The model under review builds one solid part; all positions refer to its coordinate system, in mm. Face numbers are marked on the shaded views. A direction names the side the tool comes from. Give positions to 0.01 mm unless a question says otherwise; leave off trailing zeros. Write each loop counter-clockwise with the first axis right and the second up, starting at its lowest first coordinate (ties: lowest second). Pieces come first, ordered by that corner, then holes. Notation, with made-up numbers: (60.25, -13) -> (89.25, -13) arc R18 cw to (89.25, 11) -> close; hole circle Ø4 at (76, -10). An arc over 180 degrees is marked (long way). Use CSV: the item, a comma, the result in double quotes.
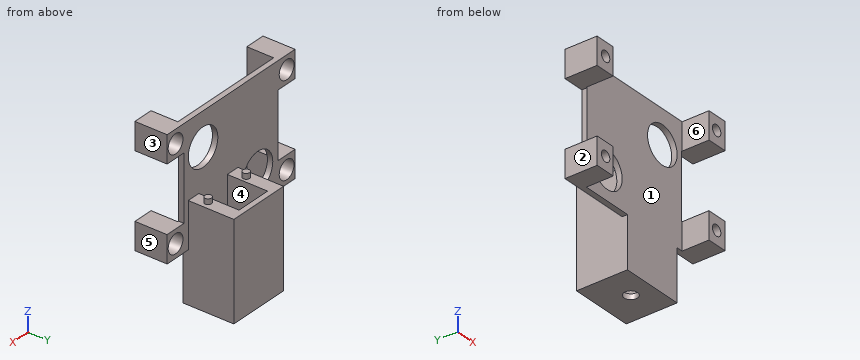
```python
from build123d import *

# Parameters (mm, degrees)
SKETCH_R        = 2
PAD_DEPTH       = 2
SKETCH001_W     = 7.6
SKETCH001_H     = 10.1
SKETCH001_R     = 2
PAD001_DEPTH    = 10
SKETCH002_R     = 7
POCKET_DEPTH    = 12.001
SKETCH004_W     = 13.5
SKETCH004_H     = 15
PAD003_DEPTH    = 34
SKETCH005_W     = 23.5
SKETCH005_H     = 19
SKETCH005_R     = 2.5
PAD004_DEPTH    = 2
SKETCH006_R     = 1.25
PAD005_DEPTH    = 2
SKETCH007_R     = 3.5
POCKET001_DEPTH = 5


with BuildPart() as part:
    # Sketch → Pad (new body)
    with BuildSketch(Plane.XZ):
        Polygon((-22.275, 22.25), (22.275, 22.25), (30.275, 22.25), (30.275, 12.15), (22.275, 12.15), (22.275, -12.15), (30.275, -12.15), (30.275, -22.25), (22.275, -22.25), (-22.275, -22.25), (-30.275, -22.25), (-30.275, -12.15), (-22.275, -12.15), (-22.275, 12.15), (-30.275, 12.15), (-30.275, 22.25), align=None)
        with Locations((-26.275, 17.2)):
            Circle(SKETCH_R, mode=Mode.SUBTRACT)
        with Locations((26.275, 17.2)):
            Circle(SKETCH_R, mode=Mode.SUBTRACT)
        with Locations((26.275, -17.2)):
            Circle(SKETCH_R, mode=Mode.SUBTRACT)
        with Locations((-26.275, -17.2)):
            Circle(SKETCH_R, mode=Mode.SUBTRACT)
    extrude(amount=PAD_DEPTH)

    # Sketch001 (on Face22 of Pad) → Pad001 (join)
    with BuildSketch(Plane.XZ.offset(2)):
        with Locations((-26.475, 17.2)):
            Rectangle(SKETCH001_W, SKETCH001_H)
        with Locations((-26.275, 17.2)):
            Circle(SKETCH001_R, mode=Mode.SUBTRACT)
        with Locations((-26.475, -17.2)):
            Rectangle(SKETCH001_W, SKETCH001_H)
        with Locations((-26.275, -17.2)):
            Circle(SKETCH001_R, mode=Mode.SUBTRACT)
        with Locations((26.475, -17.2)):
            Rectangle(SKETCH001_W, SKETCH001_H)
        with Locations((26.275, -17.2)):
            Circle(SKETCH001_R, mode=Mode.SUBTRACT)
        with Locations((26.475, 17.2)):
            Rectangle(SKETCH001_W, SKETCH001_H)
        with Locations((26.275, 17.2)):
            Circle(SKETCH001_R, mode=Mode.SUBTRACT)
    extrude(amount=PAD001_DEPTH)

    # Sketch002 (on Face4 of Pad001) → Pocket (cut, through all)
    with BuildSketch(Plane(origin=(0, 0, 0), x_dir=(-1, 0, 0), z_dir=(0, 1, 0))):
        with Locations((-13.275, 9.75)):
            Circle(SKETCH002_R)
        with Locations((12.725, -11.25)):
            Circle(SKETCH002_R)
    extrude(amount=-POCKET_DEPTH, mode=Mode.SUBTRACT)

    # Sketch004 (on DatumPlane) → Pad003 (join)
    with BuildSketch(Plane(origin=(0, 0, -5.25), x_dir=(1, 0, 0), z_dir=(0, 0, -1))):
        Polygon((-3.225, 0), (-3.225, -17), (20.275, -17), (20.275, 0), (20.275, 2), (-3.225, 2), align=None)
        with Locations((8.525, -7.5)):
            Rectangle(SKETCH004_W, SKETCH004_H, mode=Mode.SUBTRACT)
    extrude(amount=PAD003_DEPTH)

    # Sketch005 (on Face45 of Pad003) → Pad004 (join)
    with BuildSketch(Plane(origin=(0, 0, -39.25), x_dir=(1, 0, 0), z_dir=(0, 0, -1))):
        with Locations((8.525, -7.5)):
            Rectangle(SKETCH005_W, SKETCH005_H)
        with Locations((8.525, -6)):
            Circle(SKETCH005_R, mode=Mode.SUBTRACT)
    extrude(amount=PAD004_DEPTH)

    # Sketch006 (on Face16 of Pad004) → Pad005 (join)
    with BuildSketch(Plane.XY.offset(-5.25)):
        with Locations((-0.475, 5.25)):
            Circle(SKETCH006_R)
        with Locations((17.525, 5.25)):
            Circle(SKETCH006_R)
    extrude(amount=PAD005_DEPTH)

    # Sketch007 (on Face4 of Pad005) → Pocket001 (cut)
    with BuildSketch(Plane(origin=(0, 0, 0), x_dir=(-1, 0, 0), z_dir=(0, 1, 0))):
        with Locations((26.275, -17.2)):
            Circle(SKETCH007_R)
        with Locations((26.275, 17.2)):
            Circle(SKETCH007_R)
        with Locations((-26.275, 17.2)):
            Circle(SKETCH007_R)
        with Locations((-26.275, -17.2)):
            Circle(SKETCH007_R)
    extrude(amount=-POCKET001_DEPTH, mode=Mode.SUBTRACT)


solid = part.part
```
Q1. Consider section A-A (y = -7.75). Write out the cut boundary in (x, z) (3 decimals).
Derived:
outline,"(-30.275, -22.25) -> (-22.675, -22.25) -> (-22.675, -12.15) -> (-30.275, -12.15) -> close; (-30.275, 12.15) -> (-22.675, 12.15) -> (-22.675, 22.25) -> (-30.275, 22.25) -> close; (22.675, -22.25) -> (30.275, -22.25) -> (30.275, -12.15) -> (22.675, -12.15) -> close; (22.675, 12.15) -> (30.275, 12.15) -> (30.275, 22.25) -> (22.675, 22.25) -> close; hole circle Ø4 at (-26.275, -17.2); hole circle Ø4 at (-26.275, 17.2); hole circle Ø4 at (26.275, -17.2); hole circle Ø4 at (26.275, 17.2)"
Q2. Consider section B-B (z = 9.75). Write out the cut boundary in (x, y) (3 decimals), then the cut area to 3 significant figures.
Derived:
outline,"(-22.275, -2) -> (6.275, -2) -> (6.275, 0) -> (-22.275, 0) -> close; (20.275, -2) -> (22.275, -2) -> (22.275, 0) -> (20.275, 0) -> close"
area,"61.1 mm2"
Q3. Consider section C-C (z = -27.5). Write out the cut boundary in (x, y) (3 decimals), then the cut area to 3 significant figures.
Derived:
outline,"(-3.225, -2) -> (20.275, -2) -> (20.275, 17) -> (-3.225, 17) -> close; hole (1.775, 0) -> (15.275, 0) -> (15.275, 15) -> (1.775, 15) -> close"
area,"244 mm2"
Q4. The part is to be moulded in two halves that separate along X. For the marked faces 1, 2 and 3, say which applies: pulls with the +X half, pulls with the -X half, needs draft (parallel to the pull), parting line crosses it, or undercut.
Derived:
face 1,"undercut"
face 2,"pulls with the -X half"
face 3,"pulls with the +X half"
Q5. Insertion check: pin 1 (7.5 mm diameter, centred on y = 8, z = -30, fed in from -X) (3 decimals); pin 2 (3.5 mm diameter, centred on x = -25, z = 18.5, fed in from +Y); pin 3 (12 mm diameter, centred on x = -7, z = -20.5, fed in from -Y); pin 4 (3 mm diameter, centred on x = 26.275, z = 17.2, fed in from +Y). Each pin has a flat end and moves straight along its axis. Give the tip position at first contact, or say it passes through.
Derived:
pin 1,"stops at x = -3.225"
pin 2,"stops at y = 0"
pin 3,"stops at y = -2"
pin 4,"passes through"
Q6. Consider section D-D (x = -15.5). Write out the cut boundary in (y, z), then the cut area to 3 significant figures.
Derived:
outline,"(-2, -22.25) -> (0, -22.25) -> (0, -17.68) -> (-2, -17.68) -> close; (-2, -4.82) -> (0, -4.82) -> (0, 22.25) -> (-2, 22.25) -> close"
area,"63.3 mm2"
Q7. To check wall thickness, follow probe 1 along X at (y, z) = (-9.5, -17.2) (3 decimals); probe 2 along X at (y, z) = (1, -38) (3 decimals); probe 3 along Y at (x, z) = (3, -37.5). State the ranges of each line that lie inside material, in increasing order.
Derived:
probe 1,"x = -30.275 to -28.275, -24.275 to -22.675, 22.675 to 24.275, 28.275 to 30.275"
probe 2,"x = -3.225 to 1.775, 15.275 to 20.275"
probe 3,"y = -2 to 0, 15 to 17"
Q8. Machinability: for the marked faces 4, 5 and 6, which of the approach directions +Z, -Z, +X, -X, +Y, -Y give a long, thin tool a straight path to every point of the face, cutting with its end or side? Answer none if there is none.
Derived:
face 4,"+Z"
face 5,"+Z, -Z, +X, +Y, -Y"
face 6,"+Z, -Z, -Y"
